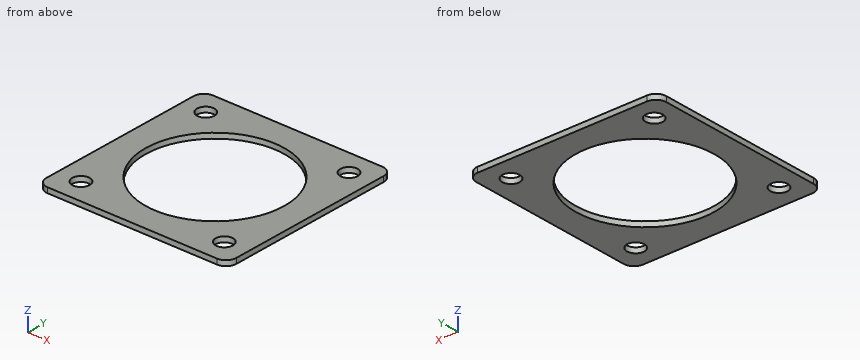
Autodesk Inventor part; units mm, degrees
ref_plane "YZ Plane" through (0, 0, 0) normal (1, 0, 0) x (0, 1, 0)
ref_plane "XZ Plane" through (0, 0, 0) normal (0, 1, 0) x (-1, 0, 0)
ref_plane "XY Plane" through (0, 0, 0) normal (0, 0, 1) x (1, 0, 0)
sketch "Sketch1" plane through (0, 0, 0) normal (0, 0, 1) x (1, 0, 0)
  line L0 (-200, 100) -> (200, 100)
  line L1 (200, 100) -> (200, -100)
  line L2 (200, -100) -> (-200, -100)
  line L3 (-200, -100) -> (-200, 100)
  line L4 (-200, 100) -> (200, -100) construction
  line L5 (200, 100) -> (-200, -100) construction
  point P0 (0, 0)
  point P1 (0, 0)
  point P2 (0, 0)
  dimension "d25" = 400
  dimension "d26" = 200
extrude "Plate1" add sketch "Sketch1" along normal blind 3
sketch "Sketch5" plane through (-197, -100, 0) normal (-1, 0, 0) x (0, -1, 0)
  line L0 (-200, 0) -> (0, 0)
  line L1 (0, 0) -> (0, 50)
  line L2 (0, 50) -> (-200, 50)
  line L3 (-200, 50) -> (-200, 0)
edge flange "Flange2" height 50 angle 90 thickness 3 bend radius 5 thickness toward (-1, 0, 0) relief round relief width 3 relief depth 1.5 corner gap 5 corner form 0 edges at (-200, 0, 3) (200, 0, 3) (0, 100, 3) (0, -100, 3) wall of the first edge with corners at (-197, 100, 0) (-197, -100, 0) (-197, -100, 50) (-197, 100, 50)
bend "Bend2"
corner "Corner2"
sketch "Sketch6" plane through (0, 0, 3) normal (0, 0, 1) x (1, 0, 0)
  circle A0 centre (-75, 0) radius 16
  circle A1 centre (75, 0) radius 16
  line L0 (0, 0) -> (0, 55.0725) construction
  circle A2 centre (33.5, 41.5) radius 5
  circle A3 centre (116.5, 41.5) radius 5
  circle A4 centre (116.5, -41.5) radius 5
  circle A5 centre (33.5, -41.5) radius 5
  line L1 (75, 0) -> (-75, 0)
  line L2 (75, 0) -> (75, -40.8866)
  circle A6 centre (-33.5, 41.5) radius 5
  circle A7 centre (-116.5, 41.5) radius 5
  circle A8 centre (-116.5, -41.5) radius 5
  circle A9 centre (-33.5, -41.5) radius 5
  point P0 (-75, -40.8866)
  dimension "d37" = 32
  dimension "d38" = 150
  dimension "d55" = 10
  dimension "d56" = 83
  dimension "d57" = 83
extrude "Cut1" cut sketch "Sketch6" against normal blind 3
sketch "Sketch7" plane through (-196.2929, 100, 8) normal (0, 1, 0) x (1, 0, 0)
  circle A0 centre (196.2929, -20) radius 6.5
  line L0 (5, 5) -> (387.5858, 5)
  line L1 (387.5858, 5) -> (388.2929, 5)
  line L2 (388.2929, 5) -> (387.5858, 5)
  line L3 (387.5858, 5) -> (5, 5)
  line L4 (5, 5) -> (4.2929, 5)
  line L5 (4.2929, 5) -> (5, 5)
  point P0 (196.2929, 8)
  dimension "d41" = 13
  dimension "d42" = 25
extrude "Extrusion2" cut sketch "Sketch7" against normal through all
pattern_linear "Rectangular Pattern1" count 3 spacing 162 along (-1, 0, 0) of "Extrusion2" first direction both ways yes
sketch "Sketch8" plane through (0, 0, 0) normal (1, 0, 0) x (0, 1, 0)
  line L0 (-96.2929, 50) -> (96.2929, 50)
  circle A0 centre (0, 28) radius 6.5
  line L1 (91.2929, 3) -> (-91.2929, 3)
  point P0 (0, 0)
  dimension "d48" = 13
  dimension "d49" = 25
extrude "Extrusion3" cut sketch "Sketch8" along normal through all both and the other way through all
pattern_linear "Rectangular Pattern2" count 3 spacing 72 along (0, 1, 0) of "Extrusion3" first direction both ways yes
sketch "Sketch9" plane through (0, 0, 0) normal (0, 0, 1) x (1, 0, 0)
  line L0 (-233.1694, -164.5287) -> (298.5547, -164.5287)
  line L1 (298.5547, -164.5287) -> (298.5547, 258.31)
  line L2 (298.5547, 258.31) -> (-233.1694, 258.31)
  line L3 (-233.1694, 258.31) -> (-233.1694, -164.5287)
  circle A0 centre (-75, 0) radius 16
  line L4 (-130, -55) -> (-20, -55)
  line L5 (-20, -55) -> (-20, 55)
  line L6 (-20, 55) -> (-130, 55)
  line L7 (-130, 55) -> (-130, -55)
  line L8 (-130, -55) -> (-20, 55) construction
  line L9 (-20, -55) -> (-130, 55) construction
  circle A1 centre (-75, 0) radius 40
  point P0 (0, 0)
  dimension "d58" = 110
  dimension "d59" = 110
  dimension "d60" = 80
extrude "Extrusion4" cut sketch "Sketch9" along normal through all both and the other way through all
fillet "Corner Round1" radius 6 4 edges at (-130, -55, 1.5) (-130, 55, 1.5) (-20, 55, 1.5) (-20, -55, 1.5)
equation "\"d25\" = Гриндер_проходная_ширина + 2 * Гриндер_размер_фланца"
equation "\"d26\" = Гриндер_высота"
equation "\"d38\" = Гриндер_Валы_между_центрами"
equation "\"d57\" = d56"
equation "\"d39\" = Thickness"
equation "\"d41\" = Гриндер_диам_отврс_корпуса"
equation "\"d42\" = Гриндер_отступ_отврс_корпуса"
equation "\"d48\" = Гриндер_диам_отврс_корпуса"
equation "\"d49\" = Гриндер_отступ_отврс_корпуса"
equation "\"d2\" = Thickness"
equation "\"d27\" = BendReliefWidth"
equation "\"d28\" = BendReliefDepth"
equation "\"d29\" = MinimumRemnant"
equation "\"d30\" = TransitionRadius"
equation "\"d33\" = BendRadius"
equation "\"d34\" = CornerReliefSize"
equation "\"d36\" = JacobiRadiusSize"
equation "\"BendReliefWidth\" = Thickness"
equation "\"BendReliefDepth\" = 0.5 * Thickness"
equation "\"CornerReliefSize\" = 4 * Thickness"
equation "\"MinimumRemnant\" = 2 * Thickness"
equation "\"TransitionRadius\" = BendRadius"
equation "\"JacobiRadiusSize\" = BendRadius"
equation "\"GapSize\" = Thickness"
equation "\"Гриндер_отступ_отврс_корпуса\" = 25"
equation "\"Гриндер_диам_отврс_корпуса\" = 13"
equation "\"Гриндер_проходная_ширина\" = 320"
equation "\"Гриндер_проходная_длина\" = 320"
equation "\"Гриндер_высота\" = 200"
equation "\"Гриндер_размер_фланца\" = 40"
equation "\"Гриндер_Валы_между_центрами\" = 150"
properties part number "NDM-VOS 161 harrow plate" material "Stainless Steel"
Input: part model. Units: mm. Frame: model coordinates. Give positions to 0.01 mm unless a question says otherwise; leave off trailing zeros. Order: outer loops, then holes, each group sorted by start corner. A loop starts at its lowest first (then second) coordinate and runs counter-clockwise, first axis right, second up. Notation, with made-up numbers: (21.25, 24) -> (33.25, 24) arc R12 cw to (33.25, 41) -> close; hole circle Ø6 at (-6.5, 1.25). An arc over 180 degrees is marked (long way). Write each question's results on one line, items separated by ' | '. Start each with the question number.
Item 1: Cut plane C-C on z = 0.75. Return the cut outline in (x, y).
Item 2: Line query: line 1 (Y direction, x = -117, z = 2.6); line 2 (X direction, y = 0, z = 0.7); line 3 (Y direction, x = -75, z = 0.8). Output: solid intervals per line, ascending.
Item 3: Cut plane A-A on y = -41.5. Return the cut outline in (x, z).
Item 4: Cut plane B-B on x = -116.5. Return the cut outline in (y, z).
Item 5: Cut plane D-D on x = -75. Return the cut outline in (y, z), then the cut area to 3 significant figures.
Established:
1) outline: (-130, -49) arc R6 ccw to (-124, -55) -> (-26, -55) arc R6 ccw to (-20, -49) -> (-20, 49) arc R6 ccw to (-26, 55) -> (-124, 55) arc R6 ccw to (-130, 49) -> close; hole circle Ø10 at (-116.5, -41.5); hole circle Ø10 at (-116.5, 41.5); hole circle Ø80 at (-75, 0); hole circle Ø10 at (-33.5, -41.5); hole circle Ø10 at (-33.5, 41.5)
2) line 1: -55 to -46.47, -36.53 to 36.53, 46.47 to 55 | line 2: -130 to -115, -35 to -20 | line 3: -55 to -40, 40 to 55
3) outline: (-130, 0) -> (-121.5, 0) -> (-121.5, 3) -> (-130, 3) -> close; (-111.5, 0) -> (-38.5, 0) -> (-38.5, 3) -> (-111.5, 3) -> close; (-28.5, 0) -> (-20, 0) -> (-20, 3) -> (-28.5, 3) -> close
4) outline: (-55, 0) -> (-46.5, 0) -> (-46.5, 3) -> (-55, 3) -> close; (-36.5, 0) -> (36.5, 0) -> (36.5, 3) -> (-36.5, 3) -> close; (46.5, 0) -> (55, 0) -> (55, 3) -> (46.5, 3) -> close
5) outline: (-55, 0) -> (-40, 0) -> (-40, 3) -> (-55, 3) -> close; (40, 0) -> (55, 0) -> (55, 3) -> (40, 3) -> close | area: 90.0 mm^2
